```python
from build123d import *

# Parameters (mm, degrees)
BASE_FLANGE1_DEPTH = 41
SKETCH2_R          = 2.5
CUT_EXTRUDE1_DEPTH = 10
SKETCH3_R          = 2.75
SKETCH3_R_2        = 2.5
CUT_EXTRUDE2_DEPTH = 10


# Sheet-metal steps are written as plain solids
with BuildPart() as part:
    # Sketch1 → Base-Flange1 (new body)
    with BuildSketch(Plane(origin=(0, 0, 0), x_dir=(1, 0, 0), z_dir=(0, 1, 0))):
        with BuildLine():
            Line((0, 0), (29.484227127, 0))
            ThreePointArc((29.484227127, 0), (29.90672353, 0.133212604), (30.176404712, 0.484667962))
            Line((30.176404712, 0.484667962), (38.681704054, 23.85278585))
            ThreePointArc((38.681704054, 23.85278585), (40.049733788, 25.635636911), (42.1929595, 26.311393382))
            Line((42.1929595, 26.311393382), (78.441184331, 26.311393382))
            ThreePointArc((78.441184331, 26.311393382), (80.843024514, 25.437195048), (82.121016981, 23.223647163))
            Line((82.121016981, 23.223647163), (84.942198964, 7.223929074))
            ThreePointArc((84.942198964, 7.223929074), (85.194131001, 6.787569985), (85.667608355, 6.615238322))
            Line((85.667608355, 6.615238322), (158.049527566, 6.615238322))
            Line((158.049527566, 6.615238322), (158.049527566, 3.615238322))
            Line((158.049527566, 3.615238322), (85.667608355, 3.615238322))
            ThreePointArc((85.667608355, 3.615238322), (83.265768172, 4.489436656), (81.987775705, 6.702984541))
            Line((81.987775705, 6.702984541), (79.166593722, 22.70270263))
            ThreePointArc((79.166593722, 22.70270263), (78.914661685, 23.139061719), (78.441184331, 23.311393382))
            Line((78.441184331, 23.311393382), (42.1929595, 23.311393382))
            ThreePointArc((42.1929595, 23.311393382), (41.770463097, 23.178180778), (41.500781916, 22.82672542))
            Line((41.500781916, 22.82672542), (32.995482574, -0.541392468))
            ThreePointArc((32.995482574, -0.541392468), (31.627452839, -2.324243529), (29.484227127, -3))
            Line((29.484227127, -3), (0, -3))
            Line((0, -3), (0, 0))
        make_face()
    extrude(amount=BASE_FLANGE1_DEPTH)

    # Sketch2 → Cut-Extrude1 (cut)
    with BuildSketch(Plane.XY.offset(3)):
        with Locations((14.991664351, 20)):
            Circle(SKETCH2_R)
    extrude(amount=-CUT_EXTRUDE1_DEPTH, mode=Mode.SUBTRACT)

    # Sketch3 → Cut-Extrude2 (cut)
    with BuildSketch(Plane.XY.offset(-3.615238322)):
        with Locations((134.991664351, 21)):
            Circle(SKETCH3_R)
        with Locations((14.991664351, 20)):
            Circle(SKETCH3_R_2)
    extrude(amount=-CUT_EXTRUDE2_DEPTH, mode=Mode.SUBTRACT)


solid = part.part
```
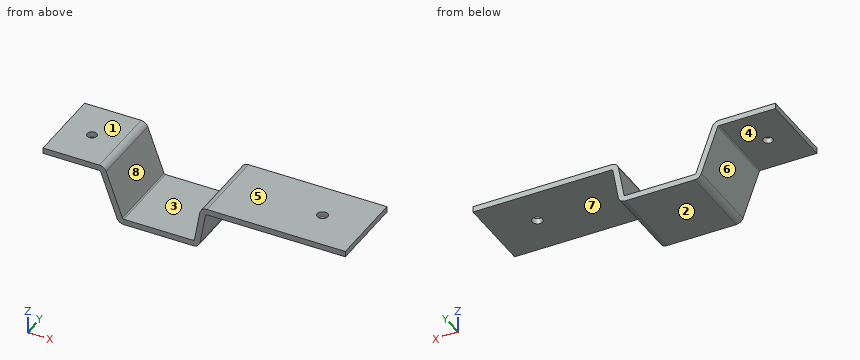
Can you work these out from the model? Positions are in its coordinate system, mm. Face numbers are marked on the shaded views. A direction names the side the tool comes from. Round coordinates to 2 decimals unless told otherwise and drop trailing zeros. Loops run counter-clockwise (first coordinate to the right, second up) from the corner with the lowest first, then second, coordinate; pieces in that order, holes last. Notation, with made-up numbers: (-21, -38.75) -> (18, -38.75) arc R15 ccw to (18, -13.75) -> close; hole circle Ø4 at (62, 12.25). An arc over 180 degrees is marked (long way). Answer in a Markdown table with one row per item.
Item 1: Suppose I cut it at B-B, the plane y = 26. List the corners of the cut face in (x, z) for me, plus the area to 3 significant figures.
Answer block:
| item | result |
|---|---|
| outline | (0, 0) -> (29.48, 0) arc R0.74 cw to (30.18, -0.48) -> (38.68, -23.85) arc R3.74 ccw to (42.19, -26.31) -> (78.44, -26.31) arc R3.74 ccw to (82.12, -23.22) -> (84.94, -7.22) arc R0.74 cw to (85.67, -6.62) -> (158.05, -6.62) -> (158.05, -3.62) -> (85.67, -3.62) arc R3.74 ccw to (81.99, -6.7) -> (79.17, -22.7) arc R0.74 cw to (78.44, -23.31) -> (42.19, -23.31) arc R0.74 cw to (41.5, -22.83) -> (33, 0.54) arc R3.74 ccw to (29.48, 3) -> (0, 3) -> close |
| area | 573 mm² |
Item 2: Will these pins go through, and if not, where does the flat tip stop? P1, Ø14.5, axis at x = 9, y = 24.5, coming from the -Z side; P2, Ø8, axis at x = 77.5, z = -4, coming from the -Y side; P3, Ø2, axis at y = 10, z = -19.5, coming from the -X side; P4, Ø18, axis at x = 62.5, y = 30.5, coming from the +Z side.
Answer block:
| item | result |
|---|---|
| P1 | z = 0 |
| P2 | through |
| P3 | x = 36.73 |
| P4 | z = -23.31 |
Item 3: Suppose I cut it at A-A, the plane z = -17.25. List the corners of the cut face in (x, y) for me.
Answer block:
| item | result |
|---|---|
| outline | (36.28, 0) -> (39.47, 0) -> (39.47, 41) -> (36.28, 41) -> close; (80.13, 0) -> (83.17, 0) -> (83.17, 41) -> (80.13, 41) -> close |
Item 4: Suppose I cut it at C-C, the plane x = 20. List the corners of the cut face in (y, z) for me.
Answer block:
| item | result |
|---|---|
| outline | (0, 0) -> (41, 0) -> (41, 3) -> (0, 3) -> close |
Item 5: We'd pull the mould along X, two halves only. Please class the marked faces 6, 7 and 8: released by +X, released by -X, zero draft, split by the parting line, or undercut.
Answer block:
| item | result |
|---|---|
| face 6 | released by -X |
| face 7 | zero draft |
| face 8 | undercut |
Item 6: If I drill on probe 1 along Z at (x, y) = (8, 19.5); probe 2 along Z at (x, y) = (109, 19); probe 3 along X at (y, z) = (33.5, -13.75), over which ranges is the centre line in solid material (lowest first)?
Answer block:
| item | result |
|---|---|
| probe 1 | 0 to 3 |
| probe 2 | -6.62 to -3.62 |
| probe 3 | 35 to 38.2, 80.75 to 83.79 |
Item 7: On a 3-axis mill with a long thin cutter (end or side, diameter ignored), from which of +Z, -Z, +X, -X, +Y, -Y can I reach the whole of each face in a straight line? I mean the marked faces 1, 2, 3, 4 and 5. Say none if no direction works.
Answer block:
| item | result |
|---|---|
| face 1 | +Z, +X, -X, +Y, -Y |
| face 2 | -Z, +X, -X, +Y, -Y |
| face 3 | +Z, +Y, -Y |
| face 4 | -Z, -X, +Y, -Y |
| face 5 | +Z, +X, +Y, -Y |
